```python
from build123d import *

# Parameters (mm, degrees)
BOSS_EXTRUDE1_DEPTH = 10
FILLET1_R           = 5.08


with BuildPart() as part:
    # Sketch1 → Boss-Extrude1 (new body)
    with BuildSketch(Plane(origin=(0, 0, 0), x_dir=(1, 0, 0), z_dir=(0, 1, 0))):
        Polygon((10, -31.75), (10, 14.429491924), (0, 31.75), (-10, 31.75), (-10, -31.75), align=None)
    extrude(amount=BOSS_EXTRUDE1_DEPTH)

    # Fillet1
    fillet1_edges = [part.edges().sort_by_distance(p)[0] for p in [
        (-10, 0, 0),
        (-5, 0, -31.75),
        (5, 0, -23.089745962),
        (10, 0, 8.660254038),
        (0, 0, 31.75),
    ]]
    fillet(fillet1_edges, radius=FILLET1_R)


solid = part.part
```
Geometry check sheet. Reference: the model listing, model coordinates, mm. Coordinates: 2 decimals unless noted, no trailing zeros. Order: outer loops, then holes, each group sorted by start corner. A loop starts at its lowest first (then second) coordinate and runs counter-clockwise, first axis right, second up.
Item 1: Section check B-B (z = -1). Enter the section's corners in (x, y), plus the area to 3 significant figures.
Item 2: Section check C-C (x = -6.25). Enter the section's corners in (y, z), plus the area to 3 significant figures.
Item 3: Section check D-D (y = 4.5). Enter the section's corners in (x, z), plus the area to 3 significant figures.
Item 4: Scan lines: line 1 along Z through (x, y) = (-0.5, 4.75); line 2 along Y through (x, z) = (-3.25, -27); line 3 along Y through (x, z) = (8.25, 11.5). Record each from-to range of solid material in increasing order.
Item 5: Section check A-A (y = 7.5). Enter the section's corners in (x, z).
Item 6: Depth check by flat-ended pin: pin 1 (1 mm diameter, centred on x = 4.5, y = 4, fed in from -Z); pin 2 (1 mm diameter, centred on x = 7.5, z = -9, fed in from -Y). Enter the tip coordinate at first touch or a pass-through.
Check sheet entries:
1. outline: (-10, 5.08) arc R5.08 ccw to (-4.92, 0) - (4.92, 0) arc R5.08 ccw to (10, 5.08) - (10, 10) - (-10, 10) - close
1. area: 189 mm2
2. outline: (0.18, -28) arc R5.08 ccw to (5.08, -31.75) - (10, -31.75) - (10, 31.75) - (5.08, 31.75) arc R5.08 ccw to (0.18, 28) - close
2. area: 614 mm2
3. outline: (-9.97, -31.72) - (-0.02, -31.72) - (9.97, -14.42) - (9.97, 31.72) - (-9.97, 31.72) - close
3. area: 1,180 mm2
4. line 1: z = -31.74 to 31.74
4. line 2: y = 0.01 to 10
4. line 3: y = 1.24 to 10
5. outline: (-10, -31.75) - (0, -31.75) - (10, -14.43) - (10, 31.75) - (-10, 31.75) - close
6. pin 1: stops at z = -24.61
6. pin 2: stops at y = 0.45
